Can you work these out from the drawing? Everything is in mm from the part's minimum corner. Coordinates: 2 decimals unless noted, no trailing zeros. Loops run counter-clockwise (first coordinate to the right, second up) from the corner with the lowest first, then second, coordinate; pieces in that order, holes last.
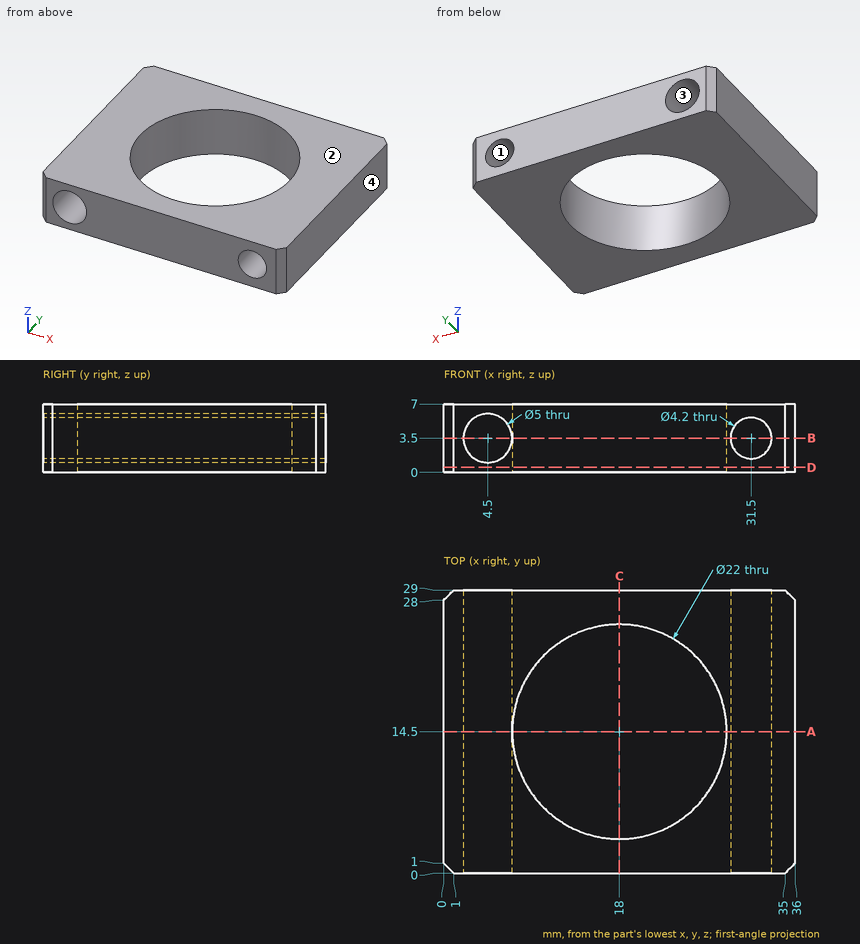
(1) I need wall thicknesses on probe 1 along Y at (x, z) = (18, 2.5); probe 2 along Z at (x, y) = (4.5, 10.5); probe 3 along X at (y, z) = (1.5, 2). Which ranges of each line are inside material? Lowest first, please.
Answers:
probe 1: y = 0 to 3.5, 25.5 to 29
probe 2: z = 0 to 1, 6 to 7
probe 3: x = 0 to 2.5, 6.5 to 30.03, 32.97 to 36
(2) Imagine slicing it at A-A, the plane y = 14.5. Write out the boundary of the cut face in (x, z), and give its area (3 significant figures).
Answers:
outline: (0, 0) - (7, 0) - (7, 7) - (0, 7) - close; (29, 0) - (36, 0) - (36, 7) - (29, 7) - close; hole circle Ø5 at (4.5, 3.5); hole circle Ø4.2 at (31.5, 3.5)
area: 64.5 mm2
(3) We'd pull the mould along Z, two halves only. Please class the marked faces 1, 2, 3 and 4: +Z half, -Z half, draft (parallel to the pull), parting line (faces both ways), or undercut.
Answers:
face 1: undercut
face 2: +Z half
face 3: undercut
face 4: draft
(4) Imagine slicing it at D-D, the plane z = 0.5. Write out the boundary of the cut face in (x, y), and give its area (3 significant figures).
Answers:
outline: (0, 1) - (1, 0) - (35, 0) - (36, 1) - (36, 28) - (35, 29) - (1, 29) - (0, 28) - close; hole circle Ø22 at (18, 14.5)
area: 662 mm2
(5) Imagine slicing it at B-B, the plane z = 3.5. Write out the boundary of the cut face in (x, y).
Answers:
outline: (0, 1) - (1, 0) - (2, 0) - (2, 29) - (1, 29) - (0, 28) - close; (7, 0) - (29.4, 0) - (29.4, 29) - (7, 29) - close; (33.6, 0) - (35, 0) - (36, 1) - (36, 28) - (35, 29) - (33.6, 29) - close; hole circle Ø22 at (18, 14.5)
(6) Imagine slicing it at C-C, the plane x = 18. Write out the boundary of the cut face in (y, z), and give its area (3 significant figures).
Answers:
outline: (0, 0) - (3.5, 0) - (3.5, 7) - (0, 7) - close; (25.5, 0) - (29, 0) - (29, 7) - (25.5, 7) - close
area: 49.0 mm2
